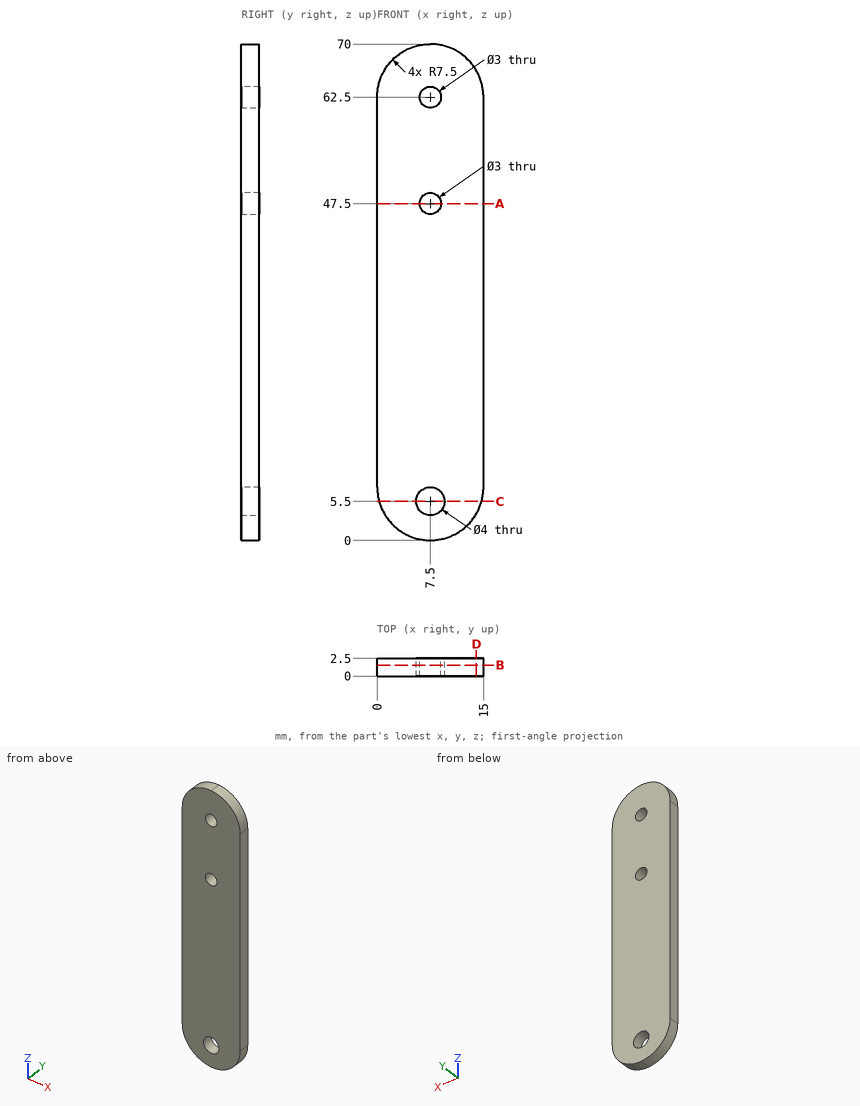
Geometry check sheet. Reference: drawing and pictorial views, mm from the part's lowest x, y, z. Coordinates: 2 decimals unless noted, no trailing zeros. Loops run counter-clockwise (first coordinate to the right, second up) from the corner with the lowest first, then second, coordinate; pieces in that order, holes last. Notation, with made-up numbers: M 11,53.5 L 29,53.5 A16 cw 29,60.5 Z; hole C 3.25,-7 d1. An arc over 180 degrees is marked long. One line per item, written item: value.
1. Section check C-C on z = 5.5. Record the cut outline in (x, y).
Answers follow:
outline: M 0.27,0 L 5.5,0 L 5.5,2.5 L 0.27,2.5 Z; M 9.5,0 L 14.73,0 L 14.73,2.5 L 9.5,2.5 Z
2. Section check D-D on x = 14. Record the cut outline in (y, z), plus the area to 3 significant figures.
Answers follow:
outline: M 0,3.76 L 2.5,3.76 L 2.5,66.24 L 0,66.24 Z
area: 156 mm^2
3. Material ranges on line 1 along X through (y, z) = (1.6, 62.5); line 2 along Z through (x, y) = (8.5, 1.3); line 3 along Z through (x, y) = (7, 1.9), recorded low to high. Write a range as from..to.
Answers follow:
line 1: 0..6, 9..15
line 2: 0.07..3.77, 7.23..46.38, 48.62..61.38, 63.62..69.93
line 3: 0.02..3.56, 7.44..46.09, 48.91..61.09, 63.91..69.98
4. Section check A-A on z = 47.5. Record the cut outline in (x, y), plus the area to 3 significant figures.
Answers follow:
outline: M 0,0 L 6,0 L 6,2.5 L 0,2.5 Z; M 9,0 L 15,0 L 15,2.5 L 9,2.5 Z
area: 30.0 mm^2
5. Section check B-B on y = 1.55. Give the number of separate pieces and of enclosed holes in the cut face, plus the area to 3 significant figures.
Answers follow:
separate pieces: 1
enclosed holes: 3
area: 975 mm^2
6. Gauge pin test, flat end, axial feed: P1, Ø1, axis at x = 10, y = 2, coming from the +Z side. Record the tip position at first contact, or that the pin passes through.
Answers follow:
P1: z = 69.73
